Study the drawing (mm; zero at the part's minimum x, y, z) and answer. Give positions to 0.01 mm unless a question says otherwise; leave off trailing zeros. Write each loop counter-clockwise with the first axis right and the second up, starting at its lowest first coordinate (ties: lowest second). Pieces come first, ordered by that corner, then holes. Notation, with made-up numbers: (32, -27) - (39, -27) arc R14 cw to (39, -17) - close; hole circle Ø3 at (20, -40). An arc over 180 degrees is marked (long way). Return JSON: item names as keys, results as strings.
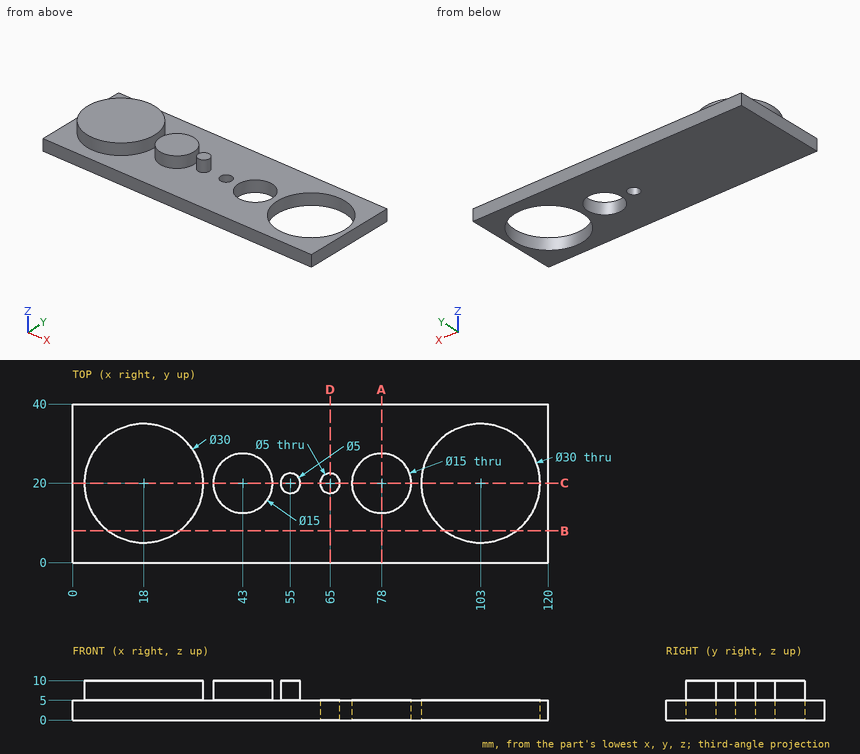
Item 1: A cutting plane is placed at B-B on y = 8. Determine the outline of the cut face in (x, z).
Answer below:
{"outline": "(0, 0) - (94, 0) - (94, 5) - (27, 5) - (27, 10) - (9, 10) - (9, 5) - (0, 5) - close; (112, 0) - (120, 0) - (120, 5) - (112, 5) - close"}
Item 2: A cutting plane is placed at A-A on x = 78. Determine the outline of the cut face in (y, z), then the cut area to 3 significant figures.
Answer below:
{"outline": "(0, 0) - (12.5, 0) - (12.5, 5) - (0, 5) - close; (27.5, 0) - (40, 0) - (40, 5) - (27.5, 5) - close", "area": "125 mm²"}
Item 3: Consider L1, parallel to Y at x = 78, z = 1.65; L2, parallel to X at y = 16, z = 4.75; L3, parallel to Y at x = 65, z = 2.8. Determine where each line is inside the solid, lowest interval first.
Answer below:
{"L1": "y = 0 to 12.5, 27.5 to 40", "L2": "x = 0 to 71.66, 84.34 to 88.54, 117.46 to 120", "L3": "y = 0 to 17.5, 22.5 to 40"}
Item 4: Flat-ended cylindrical pins translate along their axes: P1, Ø1, axis at x = 38.5, y = 9, coming from the +Z side; P2, Ø6, axis at y = 34, z = 9, coming from the +X side. Find the tip coordinate at first contact, or state that the pin passes through.
Answer below:
{"P1": "stops at z = 5", "P2": "stops at x = 28.2"}
Item 5: A cutting plane is placed at C-C on y = 20. Determine the outline of the cut face in (x, z).
Answer below:
{"outline": "(0, 0) - (62.5, 0) - (62.5, 5) - (57.5, 5) - (57.5, 10) - (52.5, 10) - (52.5, 5) - (50.5, 5) - (50.5, 10) - (35.5, 10) - (35.5, 5) - (33, 5) - (33, 10) - (3, 10) - (3, 5) - (0, 5) - close; (67.5, 0) - (70.5, 0) - (70.5, 5) - (67.5, 5) - close; (85.5, 0) - (88, 0) - (88, 5) - (85.5, 5) - close; (118, 0) - (120, 0) - (120, 5) - (118, 5) - close"}
Item 6: A cutting plane is placed at D-D on x = 65. Determine the outline of the cut face in (y, z).
Answer below:
{"outline": "(0, 0) - (17.5, 0) - (17.5, 5) - (0, 5) - close; (22.5, 0) - (40, 0) - (40, 5) - (22.5, 5) - close"}
